Design review of the part built by this model. Coordinates are the model's own, in mm. Face numbers are marked on the shaded views. Coordinates: 2 decimals unless noted, no trailing zeros. Loops run counter-clockwise (first coordinate to the right, second up) from the corner with the lowest first, then second, coordinate; pieces in that order, holes last. Notation, with made-up numbers: (45, 84.25) - (62, 84.25) arc R29 ccw to (62, 119.25) - close; hole circle Ø10 at (-21, 3.5). An arc over 180 degrees is marked (long way). Answer in a Markdown table with one row per item. Add a question column.
(1) We need section C-C, the plane z = 2.5. Write out the cut boundary in (x, y), plus the area to 3 significant figures.
(2) We need section B-B, the plane y = 29. Write out the cut boundary in (x, z), plus the area to 3 significant figures.
(3) We need section D-D, the plane y = 32. Write out the cut boundary in (x, z), plus the area to 3 significant figures.
(4) Clearance check with flat-ended pins moving along their axes: pin 1 (3.5 mm diameter, centred on x = -18.36, y = 28.67, fed in from -Z); pin 2 (8 mm diameter, centred on x = -22.5, z = 11, fed in from -Y); pin 3 (1 mm diameter, centred on y = 38.5, z = 7.5, fed in from -X); pin 4 (8 mm diameter, centred on x = -15.5, z = 9, fed in from +Y). State where each tip first meets the part, or that it passes through.
(5) To check wall thickness, follow L1, parallel to Y at x = -24.5, z = 9; L2, parallel to Z at x = -22, y = 35; L3, parallel to X at y = 39.5, z = 4.5. State the ranges of each line that lie inside material, in increasing order. Write a range as [from, to].
(6) The part is to be moulded in two halves that separate along Y. For the marked faces 1, 2, 3 and 4, say which applies: released by +Y, released by -Y, zero draft, split by the parting line, or undercut.
(7) We need section A-A, the plane x = -19.25. Write out the cut boundary in (y, z), plus the area to 3 significant figures.
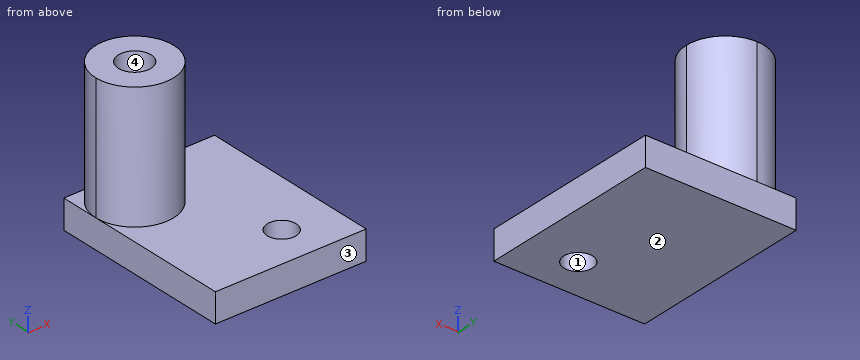
from build123d import *

# Parameters (mm, degrees)
F0_W     = 15.24
F0_H     = 18.669
F1_DEPTH = 2.921
F3_DEPTH = 12.7
F5_D     = 3.302
F5_DEPTH = 7.62
F5_TIP   = 0.992020882
F7_D     = 2.921


with BuildPart() as f1:
    # F0 (on Top) → F1 (new body)
    with BuildSketch(Plane.XY):
        with Locations((-20.8066811628, 33.9163625899)):
            Rectangle(F0_W, F0_H)
    extrude(amount=F1_DEPTH)

    # F2 (on face) → F3 (join)
    with BuildSketch(Plane.XY.offset(2.921)):
        with BuildLine():
            ThreePointArc((-28.4266811628, 39.3138625899), (-24.4896811628, 35.3768625899), (-20.5526811628, 39.3138625899))
            ThreePointArc((-20.5526811628, 39.3138625899), (-21.7058017653, 42.0977419874), (-24.4896811628, 43.2508625899))
            ThreePointArc((-24.4896811628, 43.2508625899), (-27.2735605603, 42.0977419874), (-28.4266811628, 39.3138625899))
        make_face()
    extrude(amount=F3_DEPTH)

    # F5
    with Locations(Plane.XY.offset(15.621)):
        with Locations((-24.4896811628, 39.3138625899)):
            Hole(F5_D / 2, depth=F5_DEPTH)
            with Locations((0, 0, -(F5_DEPTH + F5_TIP / 2))):  # 118° drill point
                Cone(0, F5_D / 2, F5_TIP, mode=Mode.SUBTRACT)

    # F7 (through all)
    with Locations(Plane.XY.offset(2.921)):
        with Locations((-18.3639004827, 28.6720134318)):
            Hole(F7_D / 2)


solid = f1.part
Responses:
| question | item | result |
|---|---|---|
| 1 | outline | (-28.43, 24.58) - (-13.19, 24.58) - (-13.19, 43.25) - (-28.43, 43.25) - close; hole circle Ø2.92 at (-18.36, 28.67) |
| 1 | area | 278 mm2 |
| 2 | outline | (-28.43, 0) - (-19.79, 0) - (-19.79, 2.92) - (-28.43, 2.92) - close; (-16.94, 0) - (-13.19, 0) - (-13.19, 2.92) - (-16.94, 2.92) - close |
| 2 | area | 36.2 mm2 |
| 3 | outline | (-28.43, 0) - (-13.19, 0) - (-13.19, 2.92) - (-28.43, 2.92) - close |
| 3 | area | 44.5 mm2 |
| 4 | pin 1 | stops at z = 0 |
| 4 | pin 2 | stops at y = 35.38 |
| 4 | pin 3 | stops at x = -28.41 |
| 4 | pin 4 | passes through |
| 5 | L1 | y = [35.38, 37.66], [40.96, 43.25] |
| 5 | L2 | z = [0, 2.92] |
| 5 | L3 | x = [-28.42, -20.56] |
| 6 | face 1 | undercut |
| 6 | face 2 | zero draft |
| 6 | face 3 | released by -Y |
| 6 | face 4 | undercut |
| 7 | outline | (24.58, 0) - (27.51, 0) - (27.51, 2.92) - (24.58, 2.92) - close; (29.83, 0) - (43.25, 0) - (43.25, 2.92) - (29.83, 2.92) - close |
| 7 | area | 47.7 mm2 |
